The model under review builds one solid part; all positions refer to its coordinate system, in mm. A direction names the side the tool comes from. Round coordinates to 2 decimals unless told otherwise and drop trailing zeros. Order: outer loops, then holes, each group sorted by start corner. A loop starts at its lowest first (then second) coordinate and runs counter-clockwise, first axis right, second up. Notation, with made-up numbers: M -19.75,82.5 L 34.25,82.5 A25 ccw 34.25,119.5 Z; hole C 77,-19 d10. An arc over 180 degrees is marked long. Answer as a JSON object with one key per item and string values. Group by question number.
1. Mouldability with a two-part tool opening along Z and no side actions: class faces 1 (the face through (6, -17, -68)), 2 (the face through (45, 2, -51)) as released by +Z, released by -Z, zero draft, split by the parting line, or undercut.
2. Add section B-B on x = 105. State the section outline as (y, z) points.
3. Clearance check with flat-ended pins moving along their axes: P1, Ø1.1, axis at x = 86.5, z = -7.5, coming from the -Y side; P2, Ø9, axis at x = 90, z = -67, coming from the -Y side; P3, Ø1.5, axis at x = 41, z = -42, coming from the +Y side; P4, Ø9, axis at x = 123, z = -7, coming from the -Y side. State where each tip first meets the part, or that it passes through.
4. Add section D-D on x = 91.5. Give the number of separate pieces and of enclosed holes in the cut face, and give its area (3 significant figures).
5. Machinability: for faces 3 (the face through (45.3, 1.7, -60)), 4 (the face through (29.47, -6.47, -56.543)), 5 (the face through (29.54, -2.93, -53.15)), which of the approach directions +Z, -Z, +X, -X, +Y, -Y give a long, thin tool a straight path to every point of the face, cutting with its end or side? Answer none if there is none.
6. Add section A-A on y = -21. State the section outline as (x, z) points, and give its area (3 significant figures).
7. To check wall thickness, follow probe 1 along X at (y, z) = (-11, -7); probe 2 along X at (y, z) = (1.8, -12.5); probe 3 along Z at (x, y) = (123, -12.75). State the ranges of each line that lie inside material, in increasing order. Write a range as [from, to].
```python
from build123d import *

# Parameters (mm, degrees)
ESQUISSE1_W                  = 130
ESQUISSE1_H                  = 80
BOSS_EXTRU_1_DEPTH           = 2
ESQUISSE2_W                  = 130
ESQUISSE2_H                  = 80
ESQUISSE2_R                  = 5.1
BOSS_EXTRU_2_DEPTH           = 30
ESQUISSE8_R                  = 5.5
BOSS_EXTRU_6_DEPTH           = 5
ESQUISSE3_R                  = 18
ESQUISSE3_R_2                = 5
ENL_V_MAT_EXTRU_1_DEPTH      = 31
ENL_V_MAT_EXTRU_1_DEPTH_BACK = 3
CONG_1_R                     = 1
ESQUISSE5_R                  = 5.5
ESQUISSE5_W                  = 41
ESQUISSE5_H                  = 61
ENL_V_MAT_EXTRU_2_DEPTH      = 0.5
ESQUISSE7_R                  = 2.5
BOSS_EXTRU_5_DEPTH           = 0.5
ENL_V_MAT_EXTRU_3_DEPTH      = 1
BOSS_EXTRU_8_DEPTH           = 3
CONG_2_R                     = 0.8
CONG_3_R                     = 0.8
ENL_V_MAT_EXTRU_4_DEPTH      = 3
ENL_V_MAT_EXTRU_5_DEPTH      = 17
ENL_V_MAT_EXTRU_6_DEPTH      = 17
ENL_V_MAT_EXTRU_7_DEPTH      = 11
ESQUISSE23_W                 = 8.4
ESQUISSE23_H                 = 2.6
ENL_V_MAT_EXTRU_8_DEPTH      = 11
CONG_4_R                     = 0.5


with BuildPart() as part:
    # Esquisse1 → Boss.-Extru.1 (new body)
    with BuildSketch(Plane(origin=(0, 0, 0), x_dir=(1, 0, 0), z_dir=(0, 1, 0))):
        with Locations((65, 40)):
            Rectangle(ESQUISSE1_W, ESQUISSE1_H)
    extrude(amount=BOSS_EXTRU_1_DEPTH)

    # Esquisse2 → Boss.-Extru.2 (add)
    with BuildSketch(Plane.XZ):
        with Locations((65, -40)):
            Rectangle(ESQUISSE2_W, ESQUISSE2_H)
        with Locations((123, -7)):
            Circle(ESQUISSE2_R, mode=Mode.SUBTRACT)
        with Locations((123, -73)):
            Circle(ESQUISSE2_R, mode=Mode.SUBTRACT)
        with Locations((7, -7)):
            Circle(ESQUISSE2_R, mode=Mode.SUBTRACT)
        with Locations((7, -73)):
            Circle(ESQUISSE2_R, mode=Mode.SUBTRACT)
        with BuildLine():
            Line((11.898979486, -78), (118.101020514, -78))
            ThreePointArc((118.101020514, -78), (118.050252532, -68.050252532), (128, -68.101020514))
            Line((128, -68.101020514), (128, -11.898979486))
            ThreePointArc((128, -11.898979486), (118.050252532, -11.949747468), (118.101020514, -2))
            Line((118.101020514, -2), (11.898979486, -2))
            ThreePointArc((11.898979486, -2), (11.949747468, -11.949747468), (2, -11.898979486))
            Line((2, -11.898979486), (2, -68.101020514))
            ThreePointArc((2, -68.101020514), (11.949747468, -68.050252532), (11.898979486, -78))
        make_face(mode=Mode.SUBTRACT)
    extrude(amount=BOSS_EXTRU_2_DEPTH)

    # Esquisse8 → Boss.-Extru.6 (add)
    with BuildSketch(Plane.XZ):
        with Locations((123, -7)):
            Circle(ESQUISSE8_R)
        with Locations((7, -7)):
            Circle(ESQUISSE8_R)
        with Locations((7, -73)):
            Circle(ESQUISSE8_R)
        with Locations((123, -73)):
            Circle(ESQUISSE8_R)
    extrude(amount=BOSS_EXTRU_6_DEPTH)

    # Esquisse3 → Enl_v. mat.-Extru.1 (cut, two sides)
    with BuildSketch(Plane.XZ) as enl_v_mat_extru_1_sk:
        with Locations((105, -40)):
            Circle(ESQUISSE3_R)
        with Locations((90, -67)):
            Circle(ESQUISSE3_R_2)
    extrude(amount=ENL_V_MAT_EXTRU_1_DEPTH, mode=Mode.SUBTRACT)
    extrude(enl_v_mat_extru_1_sk.sketch, amount=-ENL_V_MAT_EXTRU_1_DEPTH_BACK, mode=Mode.SUBTRACT)

    # Cong_1
    cong_1_edges = [part.edges().sort_by_distance(p)[0] for p in [
        (87, 2, -40),
    ]]
    fillet(cong_1_edges, radius=CONG_1_R)

    # Esquisse5 → Enl_v. mat.-Extru.2 (cut)
    with BuildSketch(Plane(origin=(0, 2, 0), x_dir=(1, 0, 0), z_dir=(0, 1, 0))):
        with Locations((91.5, 12.5)):
            Circle(ESQUISSE5_R)
        with Locations((45.5, 40)):
            Rectangle(ESQUISSE5_W, ESQUISSE5_H)
    extrude(amount=-ENL_V_MAT_EXTRU_2_DEPTH, mode=Mode.SUBTRACT)

    # Esquisse7 → Boss.-Extru.5 (add)
    with BuildSketch(Plane(origin=(0, 1.5, 0), x_dir=(1, 0, 0), z_dir=(0, 1, 0))):
        with Locations((45.5, 40)):
            Circle(ESQUISSE7_R)
        with BuildLine():
            Line((32.669771151, 59.088877067), (34.343279262, 56.599023537))
            ThreePointArc((34.343279262, 56.599023537), (45.5, 60), (56.656720738, 56.599023537))
            Line((56.656720738, 56.599023537), (58.330228849, 59.088877067))
            ThreePointArc((58.330228849, 59.088877067), (45.5, 63), (32.669771151, 59.088877067))
        make_face()
        with BuildLine():
            Line((38.24813152, 50.789365299), (39.921639631, 48.299511768))
            ThreePointArc((39.921639631, 48.299511768), (45.5, 50), (51.078360369, 48.299511768))
            Line((51.078360369, 48.299511768), (52.75186848, 50.789365299))
            ThreePointArc((52.75186848, 50.789365299), (45.5, 53), (38.24813152, 50.789365299))
        make_face()
        with BuildLine():
            Line((51.078360369, 31.700488232), (52.75186848, 29.210634701))
            ThreePointArc((52.75186848, 29.210634701), (45.5, 27), (38.24813152, 29.210634701))
            Line((38.24813152, 29.210634701), (39.921639631, 31.700488232))
            ThreePointArc((39.921639631, 31.700488232), (45.5, 30), (51.078360369, 31.700488232))
        make_face()
        with BuildLine():
            Line((34.343279262, 23.400976463), (32.669771151, 20.911122933))
            ThreePointArc((32.669771151, 20.911122933), (45.5, 17), (58.330228849, 20.911122933))
            Line((58.330228849, 20.911122933), (56.656720738, 23.400976463))
            ThreePointArc((56.656720738, 23.400976463), (45.5, 20), (34.343279262, 23.400976463))
        make_face()
    extrude(amount=BOSS_EXTRU_5_DEPTH)

    # Esquisse9 → Enl_v. mat.-Extru.3 (cut)
    with BuildSketch(Plane.XZ):
        with BuildLine():
            Line((78.6, -31.3), (88.673334694, -31.3))
            ThreePointArc((88.673334694, -31.3), (123.5, -40), (88.673334694, -48.7))
            Line((88.673334694, -48.7), (78.6, -48.7))
            Line((78.6, -48.7), (78.6, -31.3))
        make_face()
    extrude(amount=-ENL_V_MAT_EXTRU_3_DEPTH, mode=Mode.SUBTRACT)

    # Esquisse18 → Boss.-Extru.8 (add)
    with BuildSketch(Plane.ZY.offset(-88.5)):
        Polygon((-7.75, 0), (-4.75, 0), (-5.75, -6.5), (-6.75, -6.5), (-7.5, -5), (-6.75, -5), (-6.75, -3), (-7.75, -3), align=None)
        Polygon((-17.25, 0), (-17.25, -3), (-18.25, -3), (-18.25, -5), (-17.5, -5), (-18.25, -6.5), (-19.25, -6.5), (-20.25, 0), align=None)
    extrude(amount=BOSS_EXTRU_8_DEPTH)

    # Cong_2
    cong_2_edges = [part.edges().sort_by_distance(p)[0] for p in [
        (88.5, 0, -6.25),
        (87, 0, -4.75),
        (87, 0, -7.75),
        (85.5, 0, -6.25),
        (88.5, 0, -18.75),
        (87, 0, -17.25),
        (87, 0, -20.25),
        (85.5, 0, -18.75),
    ]]
    fillet(cong_2_edges, radius=CONG_2_R)

    # Esquisse19 → R_volution1 (revolve)
    with BuildSketch(Plane(origin=(29.5, 0, 0), x_dir=(0, 0, -1), z_dir=(1, 0, 0))):
        Polygon((55, 0), (56.85, 0), (56.85, -5), (57, -5), (56.1, -7.9), (55, -7.9), align=None)
    revolve(axis=Axis((29.5, 0, -55), (0, -1, 0)))

    # Esquisse20 → R_volution2 (revolve)
    with BuildSketch(Plane(origin=(59.5, 0, 0), x_dir=(0, 0, -1), z_dir=(1, 0, 0))):
        Polygon((18.5, 0), (20.35, 0), (20.35, -5), (20.5, -5), (19.6, -7.9), (18.5, -7.9), align=None)
    revolve(axis=Axis((59.5, 0, -18.5), (0, -1, 0)))

    # Cong_3
    cong_3_edges = [part.edges().sort_by_distance(p)[0] for p in [
        (29.5, 0, -53.15),
        (59.5, 0, -16.65),
    ]]
    fillet(cong_3_edges, radius=CONG_3_R)

    # Esquisse21 → Enl_v. mat.-Extru.4 (cut)
    with BuildSketch(Plane(origin=(29.5, 0, 0), x_dir=(0, 0, -1), z_dir=(1, 0, 0))):
        with BuildLine():
            Line((54.625, -10.5), (54.625, -0.5))
            ThreePointArc((54.625, -0.5), (55, -0.125), (55.375, -0.5))
            Line((55.375, -0.5), (55.375, -10.5))
            Line((55.375, -10.5), (54.625, -10.5))
        make_face()
    extrude(amount=-ENL_V_MAT_EXTRU_4_DEPTH, mode=Mode.SUBTRACT)

    # Esquisse21_2 → Enl_v. mat.-Extru.5 (cut)
    with BuildSketch(Plane(origin=(29.5, 0, 0), x_dir=(0, 0, -1), z_dir=(1, 0, 0))):
        with BuildLine():
            Line((54.625, -10.5), (54.625, -0.5))
            ThreePointArc((54.625, -0.5), (55, -0.125), (55.375, -0.5))
            Line((55.375, -0.5), (55.375, -10.5))
            Line((55.375, -10.5), (54.625, -10.5))
        make_face()
    extrude(amount=ENL_V_MAT_EXTRU_5_DEPTH, mode=Mode.SUBTRACT)

    # Esquisse22 → Enl_v. mat.-Extru.6 (cut)
    with BuildSketch(Plane(origin=(59.5, 0, 0), x_dir=(0, 0, -1), z_dir=(1, 0, 0))):
        with BuildLine():
            Line((18.125, -0.5), (18.125, -10.5))
            Line((18.125, -10.5), (18.875, -10.5))
            Line((18.875, -10.5), (18.875, -0.5))
            ThreePointArc((18.875, -0.5), (18.5, -0.125), (18.125, -0.5))
        make_face()
    extrude(amount=-ENL_V_MAT_EXTRU_6_DEPTH, mode=Mode.SUBTRACT)

    # Esquisse22_2 → Enl_v. mat.-Extru.7 (cut)
    with BuildSketch(Plane(origin=(59.5, 0, 0), x_dir=(0, 0, -1), z_dir=(1, 0, 0))):
        with BuildLine():
            Line((18.125, -0.5), (18.125, -10.5))
            Line((18.125, -10.5), (18.875, -10.5))
            Line((18.875, -10.5), (18.875, -0.5))
            ThreePointArc((18.875, -0.5), (18.5, -0.125), (18.125, -0.5))
        make_face()
    extrude(amount=ENL_V_MAT_EXTRU_7_DEPTH, mode=Mode.SUBTRACT)

    # Esquisse23 → Enl_v. mat.-Extru.8 (cut)
    with BuildSketch(Plane(origin=(130, 0, 0), x_dir=(0, 0, -1), z_dir=(1, 0, 0))):
        with Locations((40, -28.7)):
            Rectangle(ESQUISSE23_W, ESQUISSE23_H)
    extrude(amount=-ENL_V_MAT_EXTRU_8_DEPTH, mode=Mode.SUBTRACT)

    # Cong_4
    cong_4_edges = [part.edges().sort_by_distance(p)[0] for p in [
        (129, -27.4, -35.8),
        (129, -27.4, -44.2),
    ]]
    fillet(cong_4_edges, radius=CONG_4_R)


solid = part.part
```
Recorded:
{
 "1": {"face 1": "undercut", "face 2": "zero draft"},
 "2": {"outline": "M -30,-80 L 2,-80 L 2,-59 A1 ccw 1,-58 L 1,-58.5 L 0,-58.5 L 0,-78 L -30,-78 Z; M -30,-2 L 0,-2 L 0,-21.5 L 1,-21.5 L 1,-22 A1 ccw 2,-21 L 2,0 L -30,0 Z"},
 "3": {"P1": "stops at y = -6.1", "P2": "passes through", "P3": "stops at y = 1.5", "P4": "stops at y = -5"},
 "4": {"separate pieces": "3", "enclosed holes": "0", "area": "206 mm²"},
 "5": {"face 3": "+Y", "face 4": "-Y", "face 5": "none"},
 "6": {"outline": "M 0,-80 L 130,-80 L 130,0 L 0,0 Z; hole C 7,-73 d10.2; hole C 7,-7 d10.2; hole M 2,-68.1 A7 cw long 11.9,-78 L 118.1,-78 A7 cw long 128,-68.1 L 128,-11.9 A7 cw long 118.1,-2 L 11.9,-2 A7 cw long 2,-11.9 Z; hole C 123,-73 d10.2; hole C 123,-7 d10.2", "area": "1,010 mm²"},
 "7": {"probe 1": "x = [0, 1.9], [12.1, 14], [116, 117.9], [128.1, 130]", "probe 2": "x = [0, 25], [66, 86], [97, 130]", "probe 3": "z = [-80, -78.1], [-67.9, -66], [-14, -12.1], [-1.9, 0]"}
}
